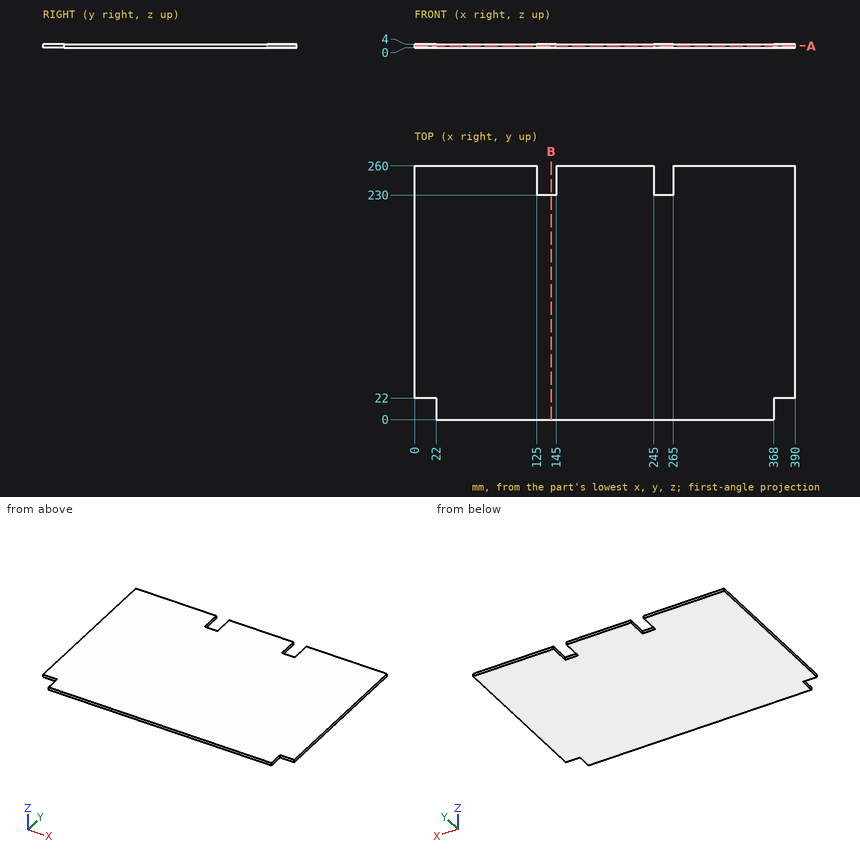
Here's the drawing with two shaded views (mm, measured from the low corner). I have some questions. Give positions to 0.01 mm unless a question says otherwise; leave off trailing zeros. Write each loop counter-clockwise with the first axis right and the second up, starting at its lowest first coordinate (ties: lowest second). Pieces come first, ordered by that corner, then holes. Notation, with made-up numbers: (63.5, -18) -> (120.5, -18) arc R18 cw to (120.5, 2) -> close; hole circle Ø9 at (-11.5, 10.25). An arc over 180 degrees is marked (long way). Use one line per item in the form item = value. Start each with the question number.
1. Imagine slicing it at B-B on x = 140. List the corners of the cut face in (y, z) for me, plus the area to 3 significant figures.
2. Imagine slicing it at A-A on z = 1.95. List the corners of the cut face in (x, y) for me, plus the area to 3 significant figures.
3. If I drill on L1, parallel to X at y = 16, z = 0.3, over which ranges is the centre line in solid material (lowest first)?
4. Will these pins go through, and if not, where does the flat tip stop? pin 1 Ø1 at (y, z) = (40, 3.5) entering from -X; pin 2 Ø1.2 at (x, z) = (253, 2) entering from +Y; pin 3 Ø1.2 at (y, z) = (14, 1.5) entering from -X; pin 4 Ø2 at (y, z) = (14, 1.5) entering from +X.
Entries:
q1.outline = (0, 0) -> (230, 0) -> (230, 4) -> (0, 4) -> close
q1.area = 920 mm²
q2.outline = (0, 22) -> (22, 22) -> (22, 0) -> (368, 0) -> (368, 22) -> (390, 22) -> (390, 260) -> (265, 260) -> (265, 230) -> (245, 230) -> (245, 260) -> (145, 260) -> (145, 230) -> (125, 230) -> (125, 260) -> (0, 260) -> close
q2.area = 99,200 mm²
q3.L1 = 22 to 368
q4.pin_1 = 0
q4.pin_2 = 230
q4.pin_3 = 22
q4.pin_4 = 368
